CAD build for the part. Positions are in the model's coordinates, mm. A direction names the side the tool comes from. Give positions to 0.01 mm unless a question says otherwise; leave off trailing zeros. Write each loop counter-clockwise with the first axis right and the second up, starting at its lowest first coordinate (ties: lowest second). Pieces come first, ordered by that corner, then holes. Notation, with made-up numbers: (-5.75, -34) - (1.25, -34) arc R23 ccw to (1.25, -6) - close; hole circle Ø8 at (53.25, -18.75). An arc over 180 degrees is marked (long way). Put each result on its own line as item: value. Start each with the question number.
1. Drop flat-ended pins along their axis: pin 1 (14.5 mm diameter, centred on x = 11.5, z = 297, fed in from -Y) (3 decimals); pin 2 (15.5 mm diameter, centred on y = -2.54, z = 889, fed in from +X) (3 decimals); pin 3 (12 mm diameter, centred on x = -15.5, y = -11, fed in from -Z); pin 4 (2.5 mm diameter, centred on x = 24, y = 3, fed in from +Z). Give the stop position or say it passes through.
2. Mould opens along X. For faces 1 (the flat face through (-22.225, -2, 451)), 2 (the flat face through (-23, 11, 914.4)), 3 (the flat face through (25.4, 0, 349)) say: +X half, -X half, draft (parallel to the pull), parting line (faces both ways), or undercut.
3. Tool access for faces 4 (the flat face through (-4, 23, 0)), 5 (the flat face through (22.225, -1, 419)): list every direction of +Z, -Z, +X, -X, +Y, -Y with a clear straight run to the whole face (end or side of a thin tool).
4. Wall check: line 1 (Z direction, x = -24, y = -2); line 2 (X direction, y = -2, z = 113.5) (3 decimals); line 3 (Y direction, x = -22.9, z = 889). Give the ranges that are in metal, low to high.
5. Cut at A-A on z = 669. List the corners of the cut face in (x, y) (3 decimals), and give its area (3 significant figures).
from build123d import *

# Parameters (mm, degrees)
F1_DEPTH = 914.4
F2_R     = 6
F3_DEPTH = 3.175
F4_W     = 47.625
F4_H     = 63.5
F5_DEPTH = 25.4
F6_R     = 6.35
F7_DEPTH = 25.4


with BuildPart() as f1:
    # F0 (on Top) → F1 (new body)
    with BuildSketch(Plane.XY):
        Polygon((22.225, -25.4), (25.4, -25.4), (25.4, 25.4), (-25.4, 25.4), (-25.4, -25.4), (-22.225, -25.4), (-22.225, 22.225), (22.225, 22.225), align=None)
    extrude(amount=F1_DEPTH)

    # F2 (on face) → F3 (cut, through all)
    with BuildSketch(Plane(origin=(-25.4, 0, 0), x_dir=(0, -1, 0), z_dir=(-1, 0, 0))):
        with Locations((2.54, 889)):
            Circle(F2_R)
    extrude(amount=-F3_DEPTH, mode=Mode.SUBTRACT)

    # F4 (on face) → F5 (cut)
    with BuildSketch(Plane.YZ.offset(25.4)):
        with Locations((-1.5875, 882.65)):
            Rectangle(F4_W, F4_H)
    extrude(amount=-F5_DEPTH, mode=Mode.SUBTRACT)

    # F6 (on face) → F7 (cut)
    with BuildSketch(Plane(origin=(0, 25.4, 0), x_dir=(-1, 0, 0), z_dir=(0, 1, 0))):
        with Locations((0, 152.4)):
            Circle(F6_R)
    extrude(amount=-F7_DEPTH, mode=Mode.SUBTRACT)


solid = f1.part
Report:
1. pin 1: stops at y = 22.225
1. pin 2: stops at x = -22.225
1. pin 3: passes through
1. pin 4: stops at z = 850.9
2. face 1: undercut
2. face 2: draft
2. face 3: +X half
3. face 4: -Z, +X, -X, +Y, -Y
3. face 5: +Z, -Z, -Y
4. line 1: z = 0 to 883.02, 894.98 to 914.4
4. line 2: x = -25.4 to -22.225, 22.225 to 25.4
4. line 3: y = -25.4 to -8.54, 3.46 to 25.4
5. outline: (-25.4, -25.4) - (-22.225, -25.4) - (-22.225, 22.225) - (22.225, 22.225) - (22.225, -25.4) - (25.4, -25.4) - (25.4, 25.4) - (-25.4, 25.4) - close
5. area: 464 mm²
